The drawing under review shows one solid part. Ordinate dimensions are in mm from its lowest x, y, z. A direction names the side the tool comes from. Give positions to 0.01 mm unless a question says otherwise; leave off trailing zeros. Write each loop counter-clockwise with the first axis right and the second up, starting at its lowest first coordinate (ties: lowest second). Pieces come first, ordered by that corner, then holes.
Q1. Insertion check: P1, Ø12, axis at x = 38.5, z = 7, coming from the -Y side; P2, Ø2, axis at x = 14, y = 42.5, coming from the -Z side (3 decimals); P3, Ø12, axis at y = 44.5, z = 13, coming from the +X side. Each pin has a flat end and moves straight along its axis. Give the tip position at first contact, or say it passes through.
Q2. Mouldability with a two-part tool opening along Y and no side actions: class the marked faces 5, 6, 7 and 8 as released by +Y, released by -Y, zero draft, split by the parting line, or undercut.
Q3. For line 1 (Z direction, x = 16.75, y = 61.15) (3 decimals); line 2 (Y direction, x = 13.5, z = 1.25); line 3 (Y direction, x = 26.5, z = 9.25), list the stretches that pass through material, from the lowest coordinate up.
Q4. We need section D-D (x = 29). Write out the cut boundary in (y, z) (3 decimals), then the cut area to 4 significant figures.
Q5. We need section B-B (y = 69). Write out the cut boundary in (x, z) (3 decimals), then the cut area to 3 significant figures.
Q6. We need section A-A (x = 15). Write out the cut boundary in (y, z) (3 decimals), then the cut area to 3 significant figures.
Q7. Machinability: for the marked faces 1, 2, 3 and 4, which of the approach directions +Z, -Z, +X, -X, +Y, -Y give a long, thin tool a straight path to every point of the face, cutting with its end or side? Answer none if there is none.
Q8. We need section C-C (y = 61.15). Write out the cut boundary in (x, z) (3 decimals).
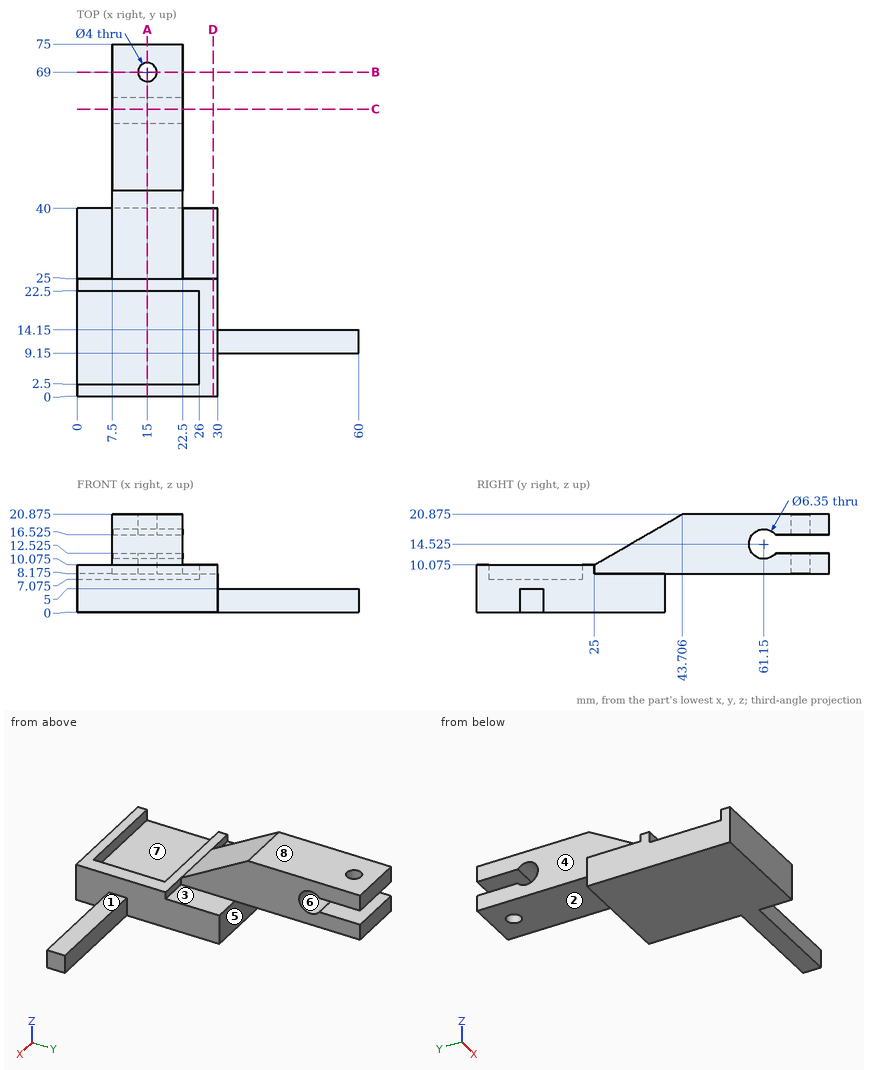
Computed:
1. P1: stops at y = 9.15
1. P2: stops at z = 8.175
1. P3: stops at x = 22.5
2. face 5: released by +Y
2. face 6: undercut
2. face 7: undercut
2. face 8: zero draft
3. line 1: z = 8.175 to 11.35, 17.7 to 20.875
3. line 2: y = 0 to 40
3. line 3: y = 0 to 25
4. outline: (0, 0) - (40, 0) - (40, 8.175) - (25, 8.175) - (25, 10.075) - (0, 10.075) - close
4. area: 374.5 mm2
5. outline: (7.5, 8.175) - (13, 8.175) - (13, 12.525) - (7.5, 12.525) - close; (7.5, 16.525) - (13, 16.525) - (13, 20.875) - (7.5, 20.875) - close; (17, 8.175) - (22.5, 8.175) - (22.5, 12.525) - (17, 12.525) - close; (17, 16.525) - (22.5, 16.525) - (22.5, 20.875) - (17, 20.875) - close
5. area: 95.7 mm2
6. outline: (0, 0) - (40, 0) - (40, 8.175) - (67, 8.175) - (67, 12.525) - (63.616, 12.525) arc R3.175 cw (long way) to (63.616, 16.525) - (67, 16.525) - (67, 20.875) - (43.706, 20.875) - (25, 10.075) - (22.5, 10.075) - (22.5, 7.075) - (2.5, 7.075) - (2.5, 10.075) - (0, 10.075) - close; (71, 8.175) - (75, 8.175) - (75, 12.525) - (71, 12.525) - close; (71, 16.525) - (75, 16.525) - (75, 20.875) - (71, 20.875) - close
6. area: 738 mm2
7. face 1: +Z, +X, +Y, -Y
7. face 2: -Z, +X, -X, +Y
7. face 3: +Z, +X, +Y
7. face 4: +Z, -X, +Y
8. outline: (7.5, 8.175) - (22.5, 8.175) - (22.5, 11.35) - (7.5, 11.35) - close; (7.5, 17.7) - (22.5, 17.7) - (22.5, 20.875) - (7.5, 20.875) - close
